from build123d import *

# Parameters (mm, degrees)
SKETCH_1_R      = 15
SKETCH_1_R_2    = 10
EXTRUDE_1_DEPTH = 15
CHAMFER_1_SIZE  = 2


with BuildPart() as part:
    # Эскиз1 → Бобышка-Вытянуть1 (new body)
    with BuildSketch(Plane.XY):
        Circle(SKETCH_1_R)
        Circle(SKETCH_1_R_2, mode=Mode.SUBTRACT)
    extrude(amount=EXTRUDE_1_DEPTH)

    # Фаска1
    chamfer_1_edges = [part.edges().sort_by_distance(p)[0] for p in [
        (-15, 0, 0),
        (-15, 0, 15),
    ]]
    chamfer(chamfer_1_edges, length=CHAMFER_1_SIZE)

    # Эскиз2 → Вырез-Повернуть1 (revolve, cut)
    with BuildSketch(Plane(origin=(0, 0, 0), x_dir=(0, 0, -1), z_dir=(1, 0, 0)), mode=Mode.PRIVATE) as cut_revolve_1_sk:
        Polygon((-7.5, 15), (-10.15, 15), (-10.15, 12), (-8.5, 10.35), (-7.5, 10.35), align=None)
    revolve(cut_revolve_1_sk.sketch.rotate(Axis((0, 0, 7.5), (0, 1, 0)), 180), axis=Axis((0, 0, 7.5), (0, 1, 0)), mode=Mode.SUBTRACT)


solid = part.part
Read the model definition and answer for the solid it produces. Units are mm, in the model's axes. A direction names the side the tool comes from. Coordinates: 2 decimals unless noted, no trailing zeros. Loops run counter-clockwise (first coordinate to the right, second up) from the corner with the lowest first, then second, coordinate; pieces in that order, holes last. Notation, with made-up numbers: (-32.5, 30) - (-24.5, 30) arc R12 cw to (-24.5, 41) - close; hole circle Ø9 at (-24, 36.25). An arc over 180 degrees is marked (long way). Answer in a Markdown table with one row per item.
Q1. Find section D-D on z = 7.5. Write down the section's boundary in (x, y).
Here are the results:
| item | result |
|---|---|
| outline | (-2.65, 12) - (-2.65, 14.76) arc R15 ccw (long way) to (2.65, 14.76) - (2.65, 12) - (1, 10.35) - (-1, 10.35) - close; hole circle Ø20 at (0, 0) |
Q2. Given P1, Ø8, axis at x = -0.5, z = 7, coming from the +Y side; P2, Ø10, axis at x = -3, y = 2, coming from the -Z side; P3, Ø5, axis at y = -8.5, z = 6.5, coming from the -X side; P4, Ø1, axis at x = 9.5, z = 2.5, coming from the +Y side, each flat-ended and moving along its own axis, determine where each tip first touches the part or whether it passes through.
Here are the results:
| item | result |
|---|---|
| P1 | stops at y = 15 |
| P2 | passes through |
| P3 | stops at x = -13.75 |
| P4 | stops at y = 12 |
Q3. Find section B-B on y = 0. Write down the section's boundary in (x, z), plus the area to 3 significant figures.
Here are the results:
| item | result |
|---|---|
| outline | (-15, 2) - (-13, 0) - (-10, 0) - (-10, 15) - (-13, 15) - (-15, 13) - close; (10, 0) - (13, 0) - (15, 2) - (15, 13) - (13, 15) - (10, 15) - close |
| area | 142 mm^2 |
Q4. For faces 5 (the cylindrical face through (1.01, 13.48, 5.05)), 6 (the cylindrical face through (-3.252, -14.643, 7.423)), determine the directions among +Z, -Z, +X, -X, +Y, -Y from which every point of the face is accessible in a straight line to the end or side of a thin tool.
Here are the results:
| item | result |
|---|---|
| face 5 | +Y |
| face 6 | +Z, -Z |
Q5. Straight lines are drawn through the part: line 1 along Y through (x, z) = (0, 11.75); line 2 along Z through (x, y) = (-0.5, 11); line 3 along X through (y, z) = (7.5, 11.5). For each, find the intervals that lie inside material, in ascending order. Write a range as [from, to].
Here are the results:
| item | result |
|---|---|
| line 1 | y = [-15, -10], [10, 15] |
| line 2 | z = [0, 5.93], [9.07, 15] |
| line 3 | x = [-12.99, -6.61], [6.61, 12.99] |
Q6. Find section A-A on x = 0. Write down the section's boundary in (y, z), plus the area to 3 significant figures.
Here are the results:
| item | result |
|---|---|
| outline | (-15, 2) - (-13, 0) - (-10, 0) - (-10, 15) - (-13, 15) - (-15, 13) - close; (10, 0) - (13, 0) - (15, 2) - (15, 4.85) - (12, 4.85) - (10.35, 6.5) - (10.35, 8.5) - (12, 10.15) - (15, 10.15) - (15, 13) - (13, 15) - (10, 15) - close |
| area | 120 mm^2 |
Q7. The mould has two halves that part along Z. Classify faces 1 (the cylindrical face through (-2.17, -9.76, 7.4)), 2 (the flat face through (7, -8, 15)), 3 (the flat face through (0, 10.35, 8)), 4 (the flat face through (7, -8, 0)): pulls with the +Z half, pulls with the -Z half, needs draft (parallel to the pull), parting line crosses it, or undercut.
Here are the results:
| item | result |
|---|---|
| face 1 | needs draft |
| face 2 | pulls with the +Z half |
| face 3 | undercut |
| face 4 | pulls with the -Z half |
Q8. Find section C-C on z = 3. Write down the section's boundary in (x, y), plus the area to 3 significant figures.
Here are the results:
| item | result |
|---|---|
| outline | circle Ø30 at (0, 0); hole circle Ø20 at (0, 0) |
| area | 393 mm^2 |
